Check sheet for the modelled part. Datum: model origin and axes. Units: mm. A direction names the side the tool comes from. Round coordinates to 2 decimals unless told otherwise and drop trailing zeros. Write each loop counter-clockwise with the first axis right and the second up, starting at its lowest first coordinate (ties: lowest second). Pieces come first, ordered by that corner, then holes. Notation, with made-up numbers: (3, 64) -> (24, 64) arc R22 cw to (24, 82) -> close; hole circle Ø4 at (71.5, -31). An arc over 180 degrees is marked (long way). Answer as a JSON object with one key per item and string values. Group by question number.
```python
from build123d import *

# Parameters (mm, degrees)
SKETCH2_R               = 7.5
CUT_EXTRUDE1_DEPTH      = 38.5
CUT_EXTRUDE1_DEPTH_BACK = 38.5
CUT_EXTRUDE2_DEPTH      = 38.500000101
CUT_EXTRUDE2_DEPTH_BACK = 38.500000101


with BuildPart() as part:
    # Sketch1 one side → Revolve1 (revolve)
    with BuildSketch(Plane(origin=(0, 0, 0), x_dir=(0, 0, -1), z_dir=(1, 0, 0))):
        with BuildLine():
            Line((-37.5, 15), (-37.5, -37.5))
            Line((-37.5, -37.5), (-32.5, -37.5))
            Line((-32.5, -37.5), (-32.5, 17.5))
            Line((-32.5, 17.5), (0, 17.5))
            Line((0, 17.5), (0, 33))
            ThreePointArc((0, 33), (-17.644049989, 34.1296112), (-35, 37.5))
            Line((-35, 37.5), (-37.5, 37.5))
            Line((-37.5, 37.5), (-37.5, 29.5))
            Line((-37.5, 29.5), (-36, 29.5))
            Line((-36, 29.5), (-36, 27))
            Line((-36, 27), (-37.5, 27))
            Line((-37.5, 27), (-37.5, 23.5))
            Line((-37.5, 23.5), (-36, 23.5))
            Line((-36, 23.5), (-36, 21))
            Line((-36, 21), (-37.5, 21))
            Line((-37.5, 21), (-37.5, 17.5))
            Line((-37.5, 17.5), (-36, 17.5))
            Line((-36, 17.5), (-36, 15))
            Line((-36, 15), (-37.5, 15))
        make_face()
    revolve(axis=Axis((0, 37.5, 0), (0, -1, 0)))

    # Sketch2 → Cut-Extrude1 (cut, two sides)
    with BuildSketch(Plane(origin=(0, 0, 0), x_dir=(0, 0, -1), z_dir=(1, 0, 0))) as cut_extrude1_sk:
        with Locations((0, -10)):
            Circle(SKETCH2_R)
    extrude(amount=CUT_EXTRUDE1_DEPTH, mode=Mode.SUBTRACT)
    extrude(cut_extrude1_sk.sketch, amount=-CUT_EXTRUDE1_DEPTH_BACK, mode=Mode.SUBTRACT)

    # Sketch3 → Cut-Extrude2 (cut, two sides)
    with BuildSketch(Plane(origin=(0, 0, 0), x_dir=(0, 0, -1), z_dir=(1, 0, 0))) as cut_extrude2_sk:
        with BuildLine():
            Line((55.2014237, -46.459477436), (54.298595824, -10))
            Line((54.298595824, -10), (25.617376915, -10))
            ThreePointArc((25.617376915, -10), (19.976616167, -11.742771762), (16.301967128, -16.363636364))
            ThreePointArc((16.301967128, -16.363636364), (0, -27.5), (-16.301967128, -16.363636364))
            ThreePointArc((-16.301967128, -16.363636364), (-19.976616167, -11.742771762), (-25.617376915, -10))
            Line((-25.617376915, -10), (-54.298595824, -10))
            Line((-54.298595824, -10), (-43.079650209, -45.071046523))
            Line((-43.079650209, -45.071046523), (55.2014237, -46.459477436))
        make_face()
    extrude(amount=CUT_EXTRUDE2_DEPTH, mode=Mode.SUBTRACT)
    extrude(cut_extrude2_sk.sketch, amount=-CUT_EXTRUDE2_DEPTH_BACK, mode=Mode.SUBTRACT)


solid = part.part
```
(1) Section check C-C on z = 0. State how many separate pieces and enclosed holes the cut face has, then the cut area to 3 significant figures.
(2) Section check D-D on y = 5. Record the cut outline in (x, z).
(3) Section check A-A on y = -13. Record the cut outline in (x, z), then the cut area to 3 significant figures.
(4) Access from +Z, -Z, +X, -X, +Y, -Y to the whole of each face (thin tool, end or side, straight path). Record for faces 4 (the flat face through (0, 17.5, 0)), 5 (the cylindrical face through (-37.18, 25.23, -4.88)), 6 (the flat face through (0, -10, 33)), 7 (the flat face through (-14, 17.5, -34)).
(5) Go/stop test with flat-tipped pins: pin 1 Ø1 at (y, z) = (-10, 20) entering from -X; pin 2 Ø9.5 at (x, z) = (0, 31) entering from -Y; pin 3 Ø24 at (y, z) = (-10, 0) entering from +X; pin 4 Ø5 at (y, z) = (11, -7) entering from -X. Record where each tip stops, or that it passes through.
(6) Release check for a two-part mould opening along Y. For faces 1 (the cylindrical face through (-28.319, -11.696, -20.046)), 2 (the cylindrical face through (-37.18, 33.44, -4.88)), 3 (the flat face through (-14, 21, 34)) record: pulls with the +Y half, pulls with the -Y half, needs draft (parallel to the pull), parting line crosses it, or undercut.
(7) Scan lines: line 1 along Y through (x, z) = (-14, 34); line 2 along Z through (x, y) = (0, -2). Record each from-to range of solid material in increasing order.
Data:
{
 "1": {"separate pieces": "3", "enclosed holes": "0", "area": "1,570 mm²"},
 "2": {"outline": "circle Ø75 at (0, 0); hole circle Ø65 at (0, 0)"},
 "3": {"outline": "(-36.86, -6.87) arc R37.5 ccw to (-32.63, -18.48) -> (-26.74, -18.48) arc R32.5 cw to (-31.76, -6.87) -> close; (-36.86, 6.87) -> (-31.76, 6.87) arc R32.5 cw to (-26.74, 18.48) -> (-32.63, 18.48) arc R37.5 ccw to start; (26.74, -18.48) -> (32.63, -18.48) arc R37.5 ccw to (36.86, -6.87) -> (31.76, -6.87) arc R32.5 cw to start; (26.74, 18.48) arc R32.5 cw to (31.76, 6.87) -> (36.86, 6.87) arc R37.5 ccw to (32.63, 18.48) -> close", "area": "251 mm²"},
 "4": {"face 4": "-Y", "face 5": "+Y, -Y", "face 6": "+Z, +X, -X, -Y", "face 7": "none"},
 "5": {"pin 1": "stops at x = -32.03", "pin 2": "stops at y = -10", "pin 3": "stops at x = 37.5", "pin 4": "stops at x = -37.23"},
 "6": {"face 1": "pulls with the -Y half", "face 2": "needs draft", "face 3": "undercut"},
 "7": {"line 1": "y = -10 to 15, 17.5 to 21, 23.5 to 27, 29.5 to 37.5", "line 2": "z = -37.5 to -32.5, 32.5 to 37.5"}
}
